CAD build for the part. Positions are in the model's coordinates, mm. Face numbers are marked on the shaded views. Give positions to 0.01 mm unless a question says otherwise; leave off trailing zeros. Loops run counter-clockwise (first coordinate to the right, second up) from the corner with the lowest first, then second, coordinate; pieces in that order, holes last.
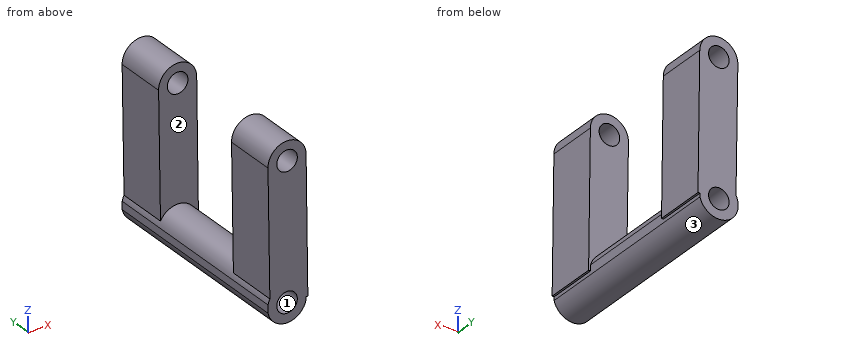
```python
from build123d import *

# Parameters (mm, degrees)
F1_DEPTH = 50
F3_DEPTH = 25
F6_D     = 10


with BuildPart() as f1:
    # F0 (on Front) → F1 (new body)
    with BuildSketch(Plane.XZ):
        with BuildLine():
            Line((-9.229952, -19.379207), (-9.229952, -23.184515))
            ThreePointArc((-9.229952, -23.184515), (-0.179062, -30.704177), (9.150997, -23.533827))
            Line((9.150997, -23.533827), (9.150997, -19.029895))
            ThreePointArc((9.150997, -19.029895), (-0.179062, -11.859545), (-9.229952, -19.379207))
        make_face()
    extrude(amount=F1_DEPTH)

    # F2 (on Front) → F3 (join)
    with BuildSketch(Plane.XZ):
        with BuildLine():
            ThreePointArc((9.257771, 43.720222), (9.258368, 43.659507), (9.258567, 43.59879))
            ThreePointArc((9.258567, 43.59879), (0.070375, 34.34049), (-9.257498, 43.458044))
            Line((-9.257498, 43.458044), (-8.264562, -21.851944))
            Line((-8.264562, -21.851944), (10.117864, -21.851944))
            Line((10.117864, -21.851944), (9.257771, 43.720222))
        make_face()
        with BuildLine():
            ThreePointArc((-9.257498, 43.458044), (0.070375, 34.34049), (9.258567, 43.59879))
            ThreePointArc((9.258567, 43.59879), (9.258368, 43.659507), (9.257771, 43.720222))
            ThreePointArc((9.257771, 43.720222), (-0.131089, 52.856429), (-9.257498, 43.458044))
        make_face()
    extrude(amount=F3_DEPTH)

    # F4: F1 across face


with BuildPart() as f1_1:
    add(f1.part)
    add(f1.part.mirror(Plane(origin=(-0.010882, -50, -21.281861), x_dir=(1, 0, 0), z_dir=(0, -1, 0))))

    # F6 (through all)
    with Locations(Plane(origin=(0, 0, 0), x_dir=(-1, 0, 0), z_dir=(0, 1, 0))):
        with Locations((0, 43.720222), (0, -21.281861)):
            Hole(F6_D / 2)


solid = f1_1.part
```
1. Saw through at C-C, the plane z = 40.5. List the corners of the cut face in (x, y), and give its area (3 significant figures).
Responses:
outline: (-9.21, -100) - (-3.82, -100) - (-3.82, -75) - (-9.21, -75) - close; (-9.21, -25) - (-3.82, -25) - (-3.82, 0) - (-9.21, 0) - close; (3.82, -100) - (9.3, -100) - (9.3, -75) - (3.82, -75) - close; (3.82, -25) - (9.3, -25) - (9.3, 0) - (3.82, 0) - close
area: 543 mm2
2. Saw through at B-B, the plane z = 14. List the corners of the cut face in (x, y), and give its area (3 significant figures).
Responses:
outline: (-8.81, -100) - (9.65, -100) - (9.65, -75) - (-8.81, -75) - close; (-8.81, -25) - (9.65, -25) - (9.65, 0) - (-8.81, 0) - close
area: 923 mm2
3. Probe line 1 along Z through (x, y) = (0, -80.75); line 2 along Y through (x, z) = (4.5, 13.5); line 3 along X through (y, z) = (-14.5, -21.5). List the from-to ranges inside material, lowest first.
Responses:
line 1: z = -30.71 to -26.28, -16.28 to 38.72, 48.72 to 52.86
line 2: y = -100 to -75, -25 to 0
line 3: x = -9.23 to -5, 5 to 10.11
4. Saw through at D-D, the plane y = -90.5. List the corners of the cut face in (x, z), and give its area (3 significant figures).
Responses:
outline: (-9.26, 43.46) - (-8.34, -16.89) arc R9.42 ccw to (-9.23, -19.38) - (-9.23, -23.18) arc R9.42 ccw to (9.15, -23.53) - (9.15, -21.85) - (10.12, -21.85) - (9.26, 43.72) arc R9.26 ccw to start; hole circle Ø10 at (0, -21.28); hole circle Ø10 at (0, 43.72)
area: 1,320 mm2
5. Drop flat-ended pins along their axis: pin 1 (8 mm diameter, centred on x = 0, z = 43.72, fed in from +Y) (3 decimals); pin 2 (4 mm diameter, centred on y = -36, z = -22, fed in from -X); pin 3 (0.5 mm diameter, centred on x = 9.5, y = -93, fed in from -Z); pin 4 (1.5 mm diameter, centred on x = 5.5, y = -49, fed in from -Z). Give the stop position or say it passes through.
Responses:
pin 1: passes through
pin 2: stops at x = -9.23
pin 3: stops at z = -21.85
pin 4: stops at z = -29.42
6. Saw through at A-A, the plane x = 0. List the corners of the cut face in (y, z).
Responses:
outline: (-100, -30.71) - (0, -30.71) - (0, -26.28) - (-100, -26.28) - close; (-100, -16.28) - (0, -16.28) - (0, 38.72) - (-25, 38.72) - (-25, -11.86) - (-75, -11.86) - (-75, 38.72) - (-100, 38.72) - close; (-100, 48.72) - (-75, 48.72) - (-75, 52.86) - (-100, 52.86) - close; (-25, 48.72) - (0, 48.72) - (0, 52.86) - (-25, 52.86) - close
7. Pull direction Z, two halves, no side cores. Call the marked faces 1, 2 and 3: released by +Z, released by -Z, zero draft, split by the parting line, or undercut.
Responses:
face 1: undercut
face 2: zero draft
face 3: released by -Z
